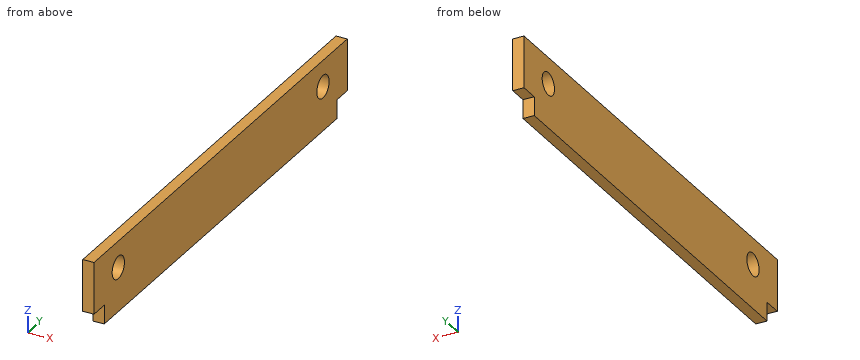
from build123d import *

# Parameters (mm, degrees)
PAD_DEPTH    = 12
SKETCH001_R  = 12
SKETCH001_W  = 20
SKETCH001_H  = 20
POCKET_DEPTH = 20


with BuildPart() as part:
    # Sketch → Pad (new body)
    with BuildSketch(Plane.YZ):
        Polygon((0, 0), (0, 75), (495, 75), (495, 0), (247.5, 0), align=None)
    extrude(amount=-PAD_DEPTH)

    # Sketch001 (on Face7 of Pad) → Pocket (cut)
    with BuildSketch(Plane(origin=(-12, 0, 0), x_dir=(0, -1, 0), z_dir=(-1, 0, 0))):
        with Locations((-447.5, 47)):
            Circle(SKETCH001_R)
        with Locations((-47.5, 47)):
            Circle(SKETCH001_R)
        with Locations((-10, 10)):
            Rectangle(SKETCH001_W, SKETCH001_H)
        with Locations((-485, 10)):
            Rectangle(SKETCH001_W, SKETCH001_H)
    extrude(amount=-POCKET_DEPTH, mode=Mode.SUBTRACT)


solid = part.part
Work out the finished part from the listing and answer in its coordinate system (mm). Give positions to 0.01 mm unless a question says otherwise; leave off trailing zeros. Loops run counter-clockwise (first coordinate to the right, second up) from the corner with the lowest first, then second, coordinate; pieces in that order, holes last. Notation, with made-up numbers: (5.5, 44.25) - (28.5, 44.25) arc R17 cw to (28.5, 51.25) - close; hole circle Ø10 at (19.5, 86). An arc over 180 degrees is marked (long way). Answer in a Markdown table with one row per item. Add a question column.
Q1. Consider line 1 along Z through (x, y) = (-5.25, 447.5); line 2 along Y through (x, z) = (-6, 52.5); line 3 along Y through (x, z) = (-6.75, 10.5). Determine where each line is inside the solid, lowest interval first.
Q2. Each of these flat-tipped pins is pushed along its axis until it touches: P1, Ø8, axis at y = 172.5, z = 38.5, coming from the +X side; P2, Ø14.5, axis at y = 447.5, z = 47, coming from the +X side; P3, Ø3.5, axis at x = -6.5, z = 13.5, coming from the +Y side; P4, Ø3.5, axis at x = -7, z = 11.5, coming from the -Y side. Where does it stop, or does it pass through?
Q3. The part is cut by section C-C (x = -6.25). Determine the outline of the cut face in (y, z).
Q4. The part is cut by section B-B (y = 47.5). Determine the outline of the cut face in (x, z).
Q5. The part is cut by section A-A (z = 47). Determine the outline of the cut face in (x, y).
Solution:
| question | item | result |
|---|---|---|
| 1 | line 1 | z = 0 to 35, 59 to 75 |
| 1 | line 2 | y = 0 to 36.83, 58.17 to 436.83, 458.17 to 495 |
| 1 | line 3 | y = 20 to 475 |
| 2 | P1 | stops at x = 0 |
| 2 | P2 | passes through |
| 2 | P3 | stops at y = 475 |
| 2 | P4 | stops at y = 20 |
| 3 | outline | (0, 20) - (20, 20) - (20, 0) - (475, 0) - (475, 20) - (495, 20) - (495, 75) - (0, 75) - close; hole circle Ø24 at (47.5, 47); hole circle Ø24 at (447.5, 47) |
| 4 | outline | (-12, 0) - (0, 0) - (0, 35) - (-12, 35) - close; (-12, 59) - (0, 59) - (0, 75) - (-12, 75) - close |
| 5 | outline | (-12, 0) - (0, 0) - (0, 35.5) - (-12, 35.5) - close; (-12, 59.5) - (0, 59.5) - (0, 435.5) - (-12, 435.5) - close; (-12, 459.5) - (0, 459.5) - (0, 495) - (-12, 495) - close |
